The listing builds one solid part. Answer for the finished solid, in the listing's coordinates (mm). Coordinates: 2 decimals unless noted, no trailing zeros. Write each loop counter-clockwise with the first axis right and the second up, starting at its lowest first coordinate (ties: lowest second). Pieces come first, ordered by that corner, then holes. Notation, with made-up numbers: M 12,11 L 39,11 A27 ccw 39,49 Z; hole C -6.5,69.5 d7. An arc over 180 degrees is marked long. Put each result on its own line as item: value. Start each with the question number.
```python
from build123d import *

# Parameters (mm, degrees)
SKETCH1_W           = 180
SKETCH1_H           = 100
SKETCH1_W_2         = 30
SKETCH1_H_2         = 8
SKETCH1_W_3         = 25
SKETCH1_H_3         = 6
BOSS_EXTRUDE1_DEPTH = 10


with BuildPart() as part:
    # Sketch1 → Boss-Extrude1 (new body)
    with BuildSketch(Plane(origin=(0, 0, 0), x_dir=(0, 0, -1), z_dir=(1, 0, 0))):
        Rectangle(SKETCH1_W, SKETCH1_H)
        Rectangle(SKETCH1_W_2, SKETCH1_H_2, mode=Mode.SUBTRACT)
        with Locations((-65, 0)):
            Rectangle(SKETCH1_W_3, SKETCH1_H_3, mode=Mode.SUBTRACT)
        with Locations((65, 0)):
            Rectangle(SKETCH1_W_3, SKETCH1_H_2, mode=Mode.SUBTRACT)
    extrude(amount=BOSS_EXTRUDE1_DEPTH)


solid = part.part
```
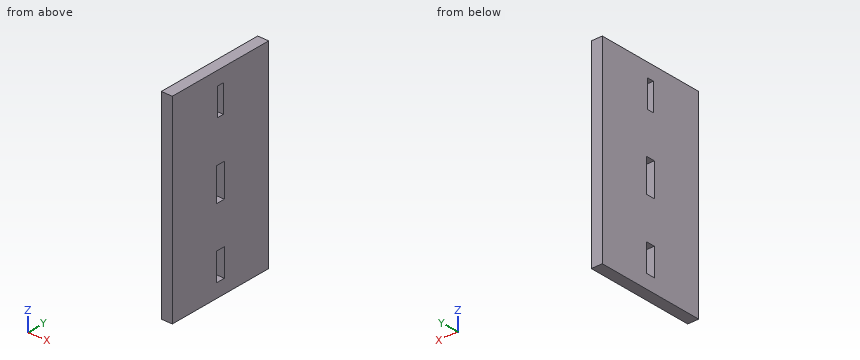
1) A cutting plane is placed at B-B on z = 8. Write down the section's boundary in (x, y).
2) Straight lines are drawn through the part: probe 1 along Z at (x, y) = (1.5, 2); probe 2 along Y at (x, z) = (6.75, 67); probe 3 along Y at (x, z) = (3.75, -66). For each, find the intervals that lie inside material, in ascending order.
3) A cutting plane is placed at A-A on x = 7. Write down the section's boundary in (y, z), then the cut area to 3 significant figures.
4) Given pin 1 Ø1.5 at (y, z) = (26.5, -21.5) entering from -X, flat-ended and moving along its own axis, determine where the tip first touches the part or whether it passes through.
Answers follow:
1. outline: M 0,-50 L 10,-50 L 10,-4 L 0,-4 Z; M 0,4 L 10,4 L 10,50 L 0,50 Z
2. probe 1: z = -90 to -77.5, -52.5 to -15, 15 to 52.5, 77.5 to 90
2. probe 2: y = -50 to -3, 3 to 50
2. probe 3: y = -50 to -4, 4 to 50
3. outline: M -50,-90 L 50,-90 L 50,90 L -50,90 Z; hole M -4,-77.5 L 4,-77.5 L 4,-52.5 L -4,-52.5 Z; hole M -4,-15 L 4,-15 L 4,15 L -4,15 Z; hole M -3,52.5 L 3,52.5 L 3,77.5 L -3,77.5 Z
3. area: 17,400 mm²
4. pin 1: stops at x = 0
